Part model, mm, in its own coordinate system. Face numbers are marked on the shaded views. A direction names the side the tool comes from. Round coordinates to 2 decimals unless told otherwise and drop trailing zeros. Loops run counter-clockwise (first coordinate to the right, second up) from the corner with the lowest first, then second, coordinate; pieces in that order, holes last.
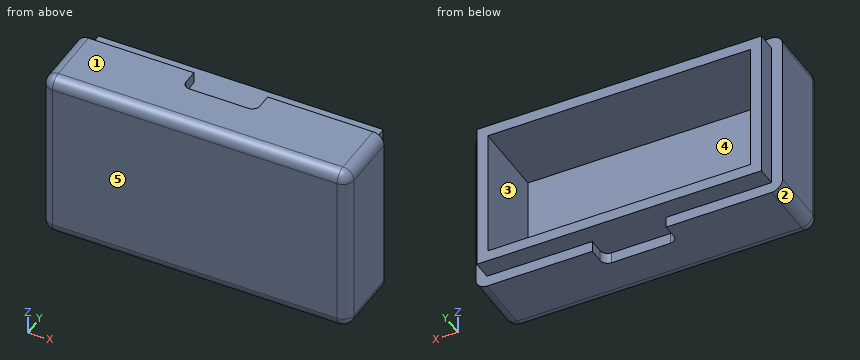
from build123d import *

# Parameters (mm, degrees)
SKETCH1_W           = 41.6
SKETCH1_H           = 23.6
BOSS_EXTRUDE1_DEPTH = 11.8
SKETCH2_W           = 35.6
SKETCH2_H           = 17.6
CUT_EXTRUDE1_DEPTH  = 10.3
SKETCH4_W           = 41.6
SKETCH4_H           = 23.6
SKETCH4_W_2         = 38.6
SKETCH4_H_2         = 20.6
CUT_EXTRUDE2_DEPTH  = 2.6
FILLET1_R           = 1.5
CUT_EXTRUDE3_DEPTH  = 1.5
CUT_EXTRUDE4_START  = -1.5
CUT_EXTRUDE4_DEPTH  = 1.5


with BuildPart() as part:
    # Sketch1 → Boss-Extrude1 (new body)
    with BuildSketch(Plane(origin=(0, 0, 0), x_dir=(1, 0, 0), z_dir=(0, 1, 0))):
        with Locations((20.8, 11.8)):
            Rectangle(SKETCH1_W, SKETCH1_H)
    extrude(amount=BOSS_EXTRUDE1_DEPTH)

    # Sketch2 → Cut-Extrude1 (cut)
    with BuildSketch(Plane(origin=(0, 11.8, 0), x_dir=(1, 0, 0), z_dir=(0, 1, 0))):
        with Locations((20.8, 11.8)):
            Rectangle(SKETCH2_W, SKETCH2_H)
    extrude(amount=-CUT_EXTRUDE1_DEPTH, mode=Mode.SUBTRACT)

    # Sketch4 → Cut-Extrude2 (cut)
    with BuildSketch(Plane(origin=(0, 11.8, 0), x_dir=(1, 0, 0), z_dir=(0, 1, 0))):
        with Locations((20.8, 11.8)):
            Rectangle(SKETCH4_W, SKETCH4_H)
        with Locations((20.8, 11.8)):
            Rectangle(SKETCH4_W_2, SKETCH4_H_2, mode=Mode.SUBTRACT)
    extrude(amount=-CUT_EXTRUDE2_DEPTH, mode=Mode.SUBTRACT)

    # Fillet1
    fillet1_edges = [part.edges().sort_by_distance(p)[0] for p in [
        (0, 4.6, -23.6),
        (41.6, 4.6, -23.6),
        (41.6, 4.6, 0),
        (0, 4.6, 0),
        (20.8, 0, -23.6),
        (41.6, 0, -11.8),
        (20.8, 0, 0),
        (0, 0, -11.8),
    ]]
    fillet(fillet1_edges, radius=FILLET1_R)

    # Sketch5 → Cut-Extrude3 (cut)
    with BuildSketch(Plane(origin=(0, 0, -23.6), x_dir=(-1, 0, 0), z_dir=(0, 0, -1))):
        with BuildLine():
            Line((-25.8, 9.2), (-15.8, 9.2))
            Line((-15.8, 9.2), (-15.8, 7.2))
            ThreePointArc((-15.8, 7.2), (-16.092893219, 6.492893219), (-16.8, 6.2))
            Line((-16.8, 6.2), (-24.8, 6.2))
            ThreePointArc((-24.8, 6.2), (-25.507106781, 6.492893219), (-25.8, 7.2))
            Line((-25.8, 7.2), (-25.8, 9.2))
        make_face()
    extrude(amount=-CUT_EXTRUDE3_DEPTH, mode=Mode.SUBTRACT)

    # Sketch6 → Cut-Extrude4 (cut)
    with BuildSketch(Plane.XY.offset(CUT_EXTRUDE4_START)):
        with BuildLine():
            Line((15.8, 9.2), (25.8, 9.2))
            Line((25.8, 9.2), (25.8, 7.2))
            ThreePointArc((25.8, 7.2), (25.507106781, 6.492893219), (24.8, 6.2))
            Line((24.8, 6.2), (16.8, 6.2))
            ThreePointArc((16.8, 6.2), (16.092893219, 6.492893219), (15.8, 7.2))
            Line((15.8, 7.2), (15.8, 9.2))
        make_face()
    extrude(amount=CUT_EXTRUDE4_DEPTH, mode=Mode.SUBTRACT)


solid = part.part
1) Drop flat-ended pins along their axis: pin 1 Ø1 at (x, z) = (9, -15.5) entering from +Y; pin 2 Ø0.8 at (y, z) = (11, -10.5) entering from +X; pin 3 Ø4.5 at (x, y) = (23, 10.5) entering from -Z. Give the stop position or say it passes through.
Values:
pin 1: stops at y = 1.5
pin 2: stops at x = 40.1
pin 3: stops at z = -22.1
2) Slice it at C-C, the plane z = -6.5. Give the cut face in (x, y).
Values:
outline: (0, 1.5) arc R1.5 ccw to (1.5, 0) - (40.1, 0) arc R1.5 ccw to (41.6, 1.5) - (41.6, 9.2) - (40.1, 9.2) - (40.1, 11.8) - (38.6, 11.8) - (38.6, 1.5) - (3, 1.5) - (3, 11.8) - (1.5, 11.8) - (1.5, 9.2) - (0, 9.2) - close
3) Slice it at A-A, the plane y = 2. Give the cut face in (x, z), then the cut area to 3 significant figures.
Values:
outline: (0, -22.1) arc R1.5 ccw to (1.5, -23.6) - (40.1, -23.6) arc R1.5 ccw to (41.6, -22.1) - (41.6, -1.5) arc R1.5 ccw to (40.1, 0) - (1.5, 0) arc R1.5 ccw to (0, -1.5) - close; hole (3, -20.6) - (38.6, -20.6) - (38.6, -3) - (3, -3) - close
area: 353 mm2
4) Mould opens along Z. For the marked faces 1, 2 and 3 say: released by +Z, released by -Z, zero draft, split by the parting line, or undercut.
Values:
face 1: released by +Z
face 2: released by -Z
face 3: undercut
5) Tool access for the marked faces 4 and 5: list every direction of +Z, -Z, +X, -X, +Y, -Y with a clear straight run to the whole face (end or side of a thin tool).
Values:
face 4: +Y
face 5: +Z, -Z, +X, -X, -Y
6) Slice it at B-B, the plane x = 20. Give the cut face in (y, z).
Values:
outline: (0, -22.1) arc R1.5 ccw to (1.5, -23.6) - (6.2, -23.6) - (6.2, -22.1) - (11.8, -22.1) - (11.8, -20.6) - (1.5, -20.6) - (1.5, -3) - (11.8, -3) - (11.8, -1.5) - (6.2, -1.5) - (6.2, 0) - (1.5, 0) arc R1.5 ccw to (0, -1.5) - close
7) Wall check: line 1 along Z through (x, y) = (9, 6.25); line 2 along Z through (x, y) = (21.5, 7.5); line 3 along X through (y, z) = (11, -12). Give the ranges that are in metal, low to high.
Values:
line 1: z = -23.6 to -20.6, -3 to 0
line 2: z = -22.1 to -20.6, -3 to -1.5
line 3: x = 1.5 to 3, 38.6 to 40.1
8) Slice it at D-D, the plane y = 8.75. Give the cut face in (x, z), then the cut area to 3 significant figures.
Values:
outline: (0, -22.1) arc R1.5 ccw to (1.5, -23.6) - (15.8, -23.6) - (15.8, -22.1) - (25.8, -22.1) - (25.8, -23.6) - (40.1, -23.6) arc R1.5 ccw to (41.6, -22.1) - (41.6, -1.5) arc R1.5 ccw to (40.1, 0) - (25.8, 0) - (25.8, -1.5) - (15.8, -1.5) - (15.8, 0) - (1.5, 0) arc R1.5 ccw to (0, -1.5) - close; hole (3, -20.6) - (38.6, -20.6) - (38.6, -3) - (3, -3) - close
area: 323 mm2
